Source: CAD feature listing. Evaluate the final solid. Frame: model axes, mm. Face numbers are marked on the shaded views. A direction names the side the tool comes from. Coordinates: 2 decimals unless noted, no trailing zeros. Order: outer loops, then holes, each group sorted by start corner. A loop starts at its lowest first (then second) coordinate and runs counter-clockwise, first axis right, second up.
```python
from build123d import *

# Parameters (mm, degrees)
SKETCH_W        = 113
SKETCH_H        = 28
SKETCH_R        = 1.6
PAD_DEPTH       = 10
SKETCH001_W     = 93.6
SKETCH001_H     = 28
SKETCH001_W_2   = 5.2
SKETCH001_H_2   = 5.2
PAD001_DEPTH    = 2
SKETCH002_W     = 3
SKETCH002_H     = 4
POCKET_DEPTH    = 113.001
SKETCH003_W     = 5.2
SKETCH003_H     = 7.2
POCKET001_DEPTH = 1


with BuildPart() as part:
    # Sketch → Pad (new body)
    with BuildSketch(Plane.XY):
        with Locations((41.5, 7)):
            Rectangle(SKETCH_W, SKETCH_H)
        Circle(SKETCH_R, mode=Mode.SUBTRACT)
        with Locations((0, 14)):
            Circle(SKETCH_R, mode=Mode.SUBTRACT)
        with Locations((16.6, 0)):
            Circle(SKETCH_R, mode=Mode.SUBTRACT)
        with Locations((16.6, 14)):
            Circle(SKETCH_R, mode=Mode.SUBTRACT)
        with Locations((33.2, 0)):
            Circle(SKETCH_R, mode=Mode.SUBTRACT)
        with Locations((33.2, 14)):
            Circle(SKETCH_R, mode=Mode.SUBTRACT)
        with Locations((49.8, 0)):
            Circle(SKETCH_R, mode=Mode.SUBTRACT)
        with Locations((49.8, 14)):
            Circle(SKETCH_R, mode=Mode.SUBTRACT)
        with Locations((66.4, 0)):
            Circle(SKETCH_R, mode=Mode.SUBTRACT)
        with Locations((66.4, 14)):
            Circle(SKETCH_R, mode=Mode.SUBTRACT)
        with Locations((83, 0)):
            Circle(SKETCH_R, mode=Mode.SUBTRACT)
        with Locations((83, 14)):
            Circle(SKETCH_R, mode=Mode.SUBTRACT)
    extrude(amount=PAD_DEPTH)

    # Sketch001 → Pad001 (join)
    with BuildSketch(Plane.XY):
        with Locations((41.5, 7)):
            Rectangle(SKETCH001_W, SKETCH001_H)
        Rectangle(SKETCH001_W_2, SKETCH001_H_2, mode=Mode.SUBTRACT)
        with Locations((0, 14)):
            Rectangle(SKETCH001_W_2, SKETCH001_H_2, mode=Mode.SUBTRACT)
        with Locations((16.6, 0)):
            Rectangle(SKETCH001_W_2, SKETCH001_H_2, mode=Mode.SUBTRACT)
        with Locations((16.6, 14)):
            Rectangle(SKETCH001_W_2, SKETCH001_H_2, mode=Mode.SUBTRACT)
        with Locations((33.2, 0)):
            Rectangle(SKETCH001_W_2, SKETCH001_H_2, mode=Mode.SUBTRACT)
        with Locations((33.2, 14)):
            Rectangle(SKETCH001_W_2, SKETCH001_H_2, mode=Mode.SUBTRACT)
        with Locations((49.8, 0)):
            Rectangle(SKETCH001_W_2, SKETCH001_H_2, mode=Mode.SUBTRACT)
        with Locations((49.8, 14)):
            Rectangle(SKETCH001_W_2, SKETCH001_H_2, mode=Mode.SUBTRACT)
        with Locations((66.4, 0)):
            Rectangle(SKETCH001_W_2, SKETCH001_H_2, mode=Mode.SUBTRACT)
        with Locations((66.4, 14)):
            Rectangle(SKETCH001_W_2, SKETCH001_H_2, mode=Mode.SUBTRACT)
        with Locations((83, 0)):
            Rectangle(SKETCH001_W_2, SKETCH001_H_2, mode=Mode.SUBTRACT)
        with Locations((83, 14)):
            Rectangle(SKETCH001_W_2, SKETCH001_H_2, mode=Mode.SUBTRACT)
    extrude(amount=-PAD001_DEPTH)

    # Sketch002 (on Face2 of Pad001) → Pocket (cut, through all)
    with BuildSketch(Plane(origin=(-15, 0, 0), x_dir=(0, -1, 0), z_dir=(-1, 0, 0))):
        with Locations((-19.5, 5)):
            Rectangle(SKETCH002_W, SKETCH002_H)
        with Locations((5.5, 5)):
            Rectangle(SKETCH002_W, SKETCH002_H)
    extrude(amount=-POCKET_DEPTH, mode=Mode.SUBTRACT)

    # Sketch003 → Pocket001 (cut)
    with BuildSketch(Plane.XY.offset(-2)):
        Rectangle(SKETCH003_W, SKETCH003_H)
        with Locations((0, 14)):
            Rectangle(SKETCH003_W, SKETCH003_H)
        with Locations((16.6, 0)):
            Rectangle(SKETCH003_W, SKETCH003_H)
        with Locations((16.6, 14)):
            Rectangle(SKETCH003_W, SKETCH003_H)
        with Locations((33.2, 0)):
            Rectangle(SKETCH003_W, SKETCH003_H)
        with Locations((33.2, 14)):
            Rectangle(SKETCH003_W, SKETCH003_H)
        with Locations((49.8, 0)):
            Rectangle(SKETCH003_W, SKETCH003_H)
        with Locations((49.8, 14)):
            Rectangle(SKETCH003_W, SKETCH003_H)
        with Locations((66.4, 0)):
            Rectangle(SKETCH003_W, SKETCH003_H)
        with Locations((66.4, 14)):
            Rectangle(SKETCH003_W, SKETCH003_H)
        with Locations((83, 0)):
            Rectangle(SKETCH003_W, SKETCH003_H)
        with Locations((83, 14)):
            Rectangle(SKETCH003_W, SKETCH003_H)
    extrude(amount=POCKET001_DEPTH, mode=Mode.SUBTRACT)


solid = part.part
```
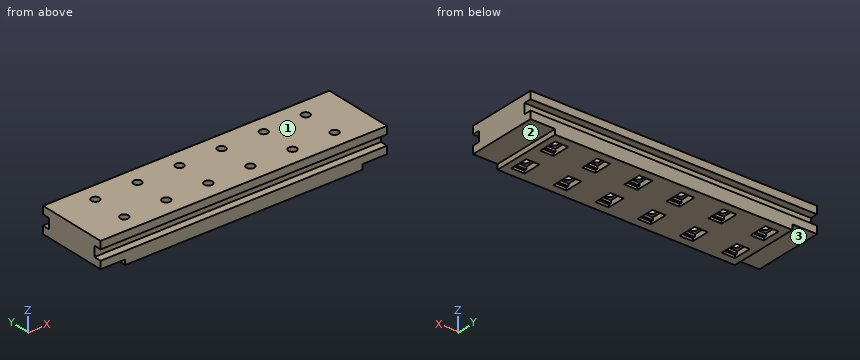
1. Section query B-B, the plane x = 75. Output: boundary loops of the cut face in (y, z), plus the area to 3 significant figures.
2. Material intervals for line 1 along Y through (x, z) = (16.6, 6); line 2 along Y through (x, z) = (83, 7.25); line 3 along X through (y, z) = (4.75, -1.5), sorted ascending.
3. Contact query for flat-ended pins moving along their axis: P1, Ø2.5, axis at x = 48.5, y = 0.5, coming from the -Z side; P2, Ø1.1, axis at x = 48.5, y = 11, coming from the -Z side; P3, Ø1.6, axis at y = 13.5, z = -1, coming from the -X side. Output: stop coordinate, or through.
4. Section query A-A, the plane z = 2. Count the separate pieces of the cut face and the enclosed holes in it, plus the area to 3 significant figures.
5. Section query C-C, the plane y = 6.75. Output: boundary loops of the cut face in (x, z).
6. Access query for the marked faces 1, 2 and 3. Directions: +Z, -Z, +X, -X, +Y, -Y. A direction counts if a zero-diameter tool reaches every point of the face in a straight line with its end or side. Return the directions, or none.
Answer key:
1. outline: (-7, -2) - (21, -2) - (21, 3) - (18, 3) - (18, 7) - (21, 7) - (21, 10) - (-7, 10) - (-7, 7) - (-4, 7) - (-4, 3) - (-7, 3) - close
1. area: 312 mm2
2. line 1: y = -4 to -1.6, 1.6 to 12.4, 15.6 to 18
2. line 2: y = -7 to -1.6, 1.6 to 12.4, 15.6 to 21
2. line 3: x = -5.3 to 88.3
3. P1: stops at z = 0
3. P2: stops at z = -1
3. P3: stops at x = -5.3
4. separate pieces: 1
4. enclosed holes: 12
4. area: 3,070 mm2
5. outline: (-15, 0) - (-5.3, 0) - (-5.3, -2) - (88.3, -2) - (88.3, 0) - (98, 0) - (98, 10) - (-15, 10) - close
6. face 1: +Z, +X, -X, +Y, -Y
6. face 2: -Z, +X, +Y, -Y
6. face 3: -Z, -X, +Y, -Y
